The figure shows three views and two pictorial views of one solid part (mm, origin at its lowest corner). Answer the questions. Coordinates: 2 decimals unless noted, no trailing zeros. Write each loop counter-clockwise with the first axis right and the second up, starting at its lowest first coordinate (ties: lowest second). Pieces come first, ordered by that corner, then holes.
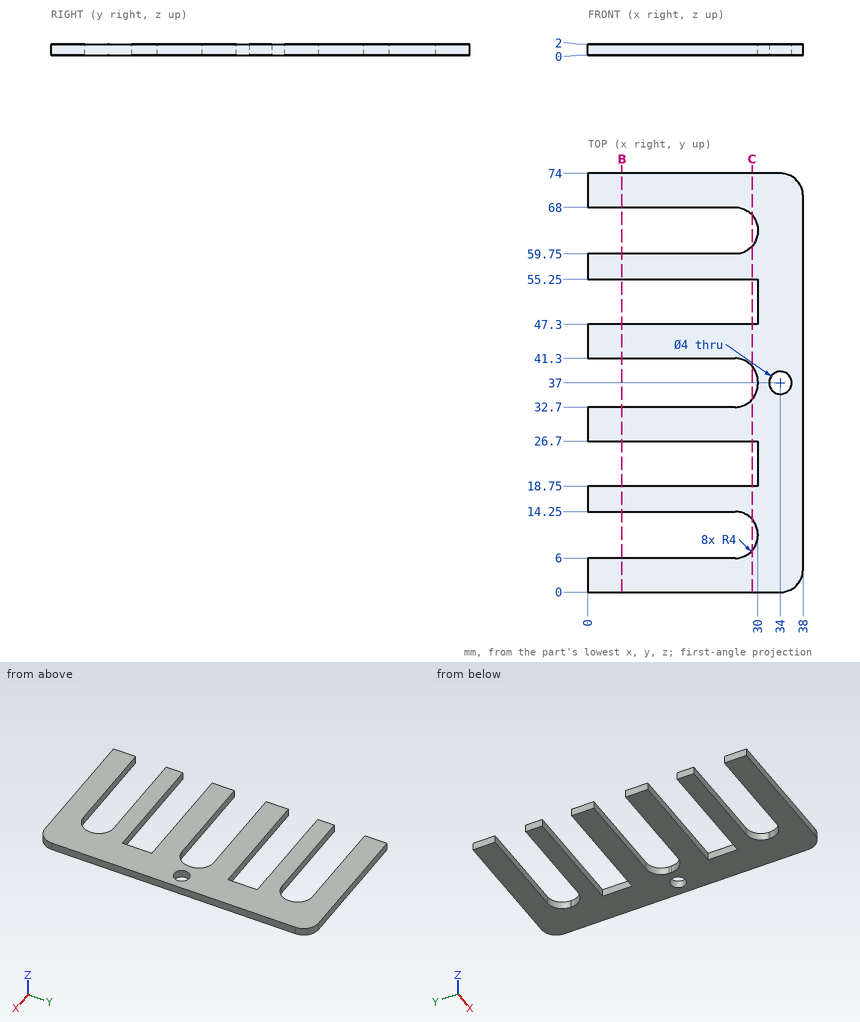
Item 1: The part is cut by section B-B (x = 6). Give the vertices of the cut face in (y, z).
Item 2: Find the intervals of material crossed by probe 1 along Y at (x, z) = (16, 0.1); probe 2 along Y at (x, z) = (34, 1.25); probe 3 along Y at (x, z) = (27, 0.75), in increasing order.
Item 3: The part is cut by section C-C (x = 29). Give the vertices of the cut face in (y, z).
Answer:
1. outline: (0, 0) - (6, 0) - (6, 2) - (0, 2) - close; (14.25, 0) - (18.75, 0) - (18.75, 2) - (14.25, 2) - close; (26.7, 0) - (32.7, 0) - (32.7, 2) - (26.7, 2) - close; (41.3, 0) - (47.3, 0) - (47.3, 2) - (41.3, 2) - close; (55.25, 0) - (59.75, 0) - (59.75, 2) - (55.25, 2) - close; (68, 0) - (74, 0) - (74, 2) - (68, 2) - close
2. probe 1: y = 0 to 6, 14.25 to 18.75, 26.7 to 32.7, 41.3 to 47.3, 55.25 to 59.75, 68 to 74
2. probe 2: y = 0 to 35, 39 to 74
2. probe 3: y = 0 to 6.13, 14.12 to 18.75, 26.7 to 32.83, 41.17 to 47.3, 55.25 to 59.88, 67.87 to 74
3. outline: (0, 0) - (7.35, 0) - (7.35, 2) - (0, 2) - close; (12.9, 0) - (18.75, 0) - (18.75, 2) - (12.9, 2) - close; (26.7, 0) - (34.05, 0) - (34.05, 2) - (26.7, 2) - close; (39.95, 0) - (47.3, 0) - (47.3, 2) - (39.95, 2) - close; (55.25, 0) - (61.1, 0) - (61.1, 2) - (55.25, 2) - close; (66.65, 0) - (74, 0) - (74, 2) - (66.65, 2) - close
